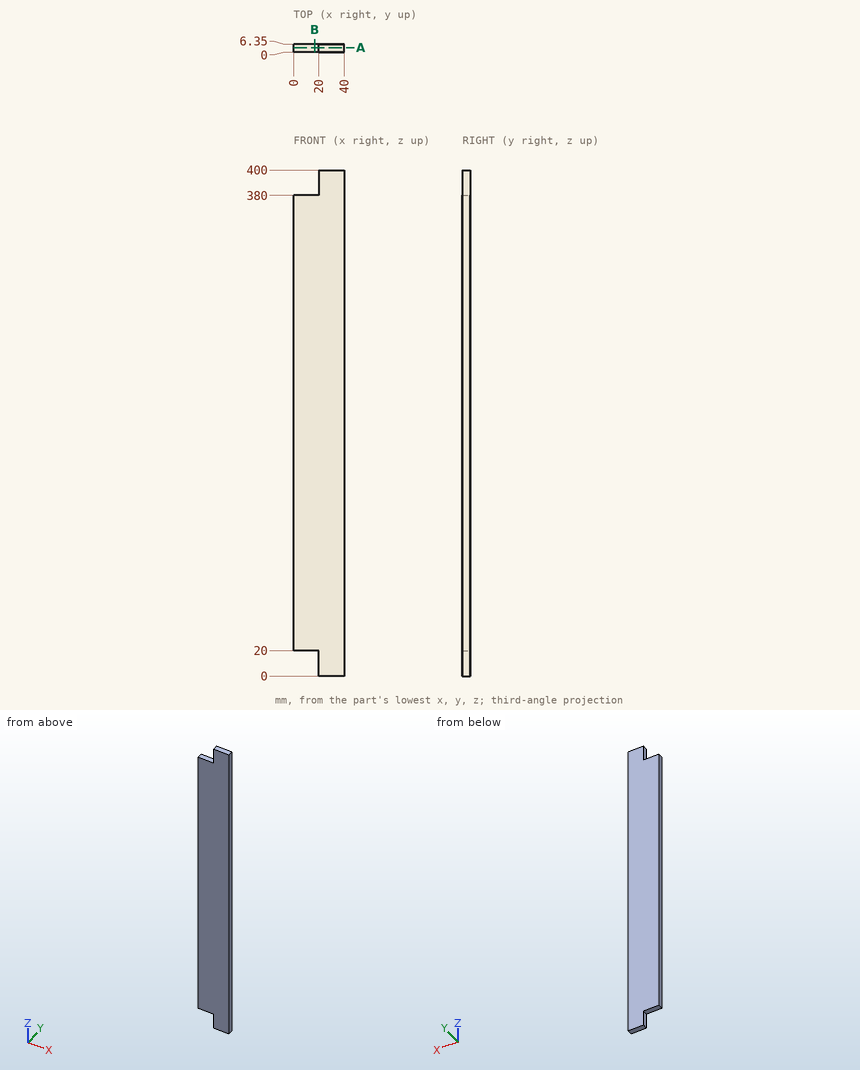
Study the drawing (mm; zero at the part's minimum x, y, z) and answer. Coordinates: 2 decimals unless noted, no trailing zeros. Loops run counter-clockwise (first coordinate to the right, second up) from the corner with the lowest first, then second, coordinate; pieces in that order, holes last. Notation, with made-up numbers: (-34, 78.25) -> (11, 78.25) arc R25 cw to (11, 91.25) -> close; hole circle Ø6 at (66.25, 49). An arc over 180 degrees is marked (long way). Write item = value, one per line. Start each with the question number.
1) Given P1, Ø3, axis at y = 2.5, z = 391.5, coming from the -X side; P2, Ø3, axis at x = 14.5, y = 1, coming from the -Z side, each flat-ended and moving along its own axis, determine where each tip first touches the part or whether it passes through.
2) The part is cut by section A-A, the plane y = 3.5. Determine the outline of the cut face in (x, z), plus the area to 3 significant figures.
3) The part is cut by section B-B, the plane x = 16.5. Determine the outline of the cut face in (y, z).
4) Find the intervals of material crossed by L1, parallel to Z at x = 17, y = 3.75; L2, parallel to X at y = 2, z = 18, in increasing order. Write a range as from..to.
Result:
q1.P1 = 20
q1.P2 = 20
q2.outline = (0, 20) -> (20, 20) -> (20, 0) -> (40, 0) -> (40, 400) -> (20, 400) -> (20, 380) -> (0, 380) -> close
q2.area = 15,200 mm²
q3.outline = (0, 20) -> (6.35, 20) -> (6.35, 380) -> (0, 380) -> close
q4.L1 = 20..380
q4.L2 = 20..40
